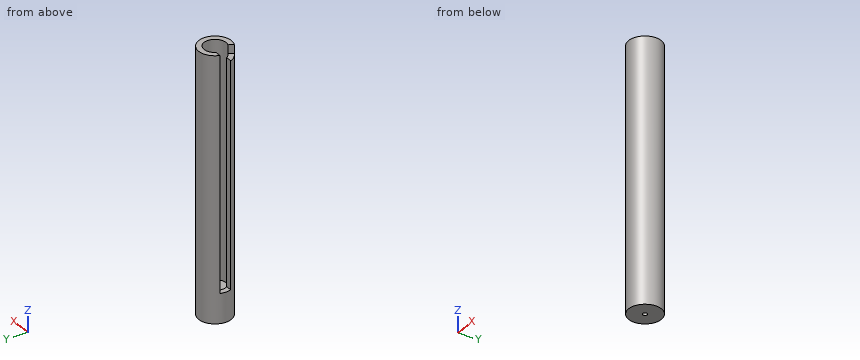
from build123d import *

# Parameters (mm, degrees)
SKETCH1_R           = 19.05
BOSS_EXTRUDE1_DEPTH = 304.8
SKETCH3_R           = 12.7
CUT_EXTRUDE1_DEPTH  = 273.05
SKETCH4_R           = 2.54
CUT_EXTRUDE2_DEPTH  = 31.75
CUT_EXTRUDE3_DEPTH  = 273.05
CUT_EXTRUDE4_DEPTH  = 12.7


with BuildPart() as part:
    # Sketch1 → Boss-Extrude1 (new body)
    with BuildSketch(Plane.XY):
        Circle(SKETCH1_R)
    extrude(amount=BOSS_EXTRUDE1_DEPTH)

    # Sketch3 → Cut-Extrude1 (cut)
    with BuildSketch(Plane.XY.offset(304.8)):
        Circle(SKETCH3_R)
    extrude(amount=-CUT_EXTRUDE1_DEPTH, mode=Mode.SUBTRACT)

    # Sketch4 → Cut-Extrude2 (cut)
    with BuildSketch(Plane(origin=(0, 0, 0), x_dir=(-1, 0, 0), z_dir=(0, 0, -1))):
        Circle(SKETCH4_R)
    extrude(amount=-CUT_EXTRUDE2_DEPTH, mode=Mode.SUBTRACT)

    # Sketch5 → Cut-Extrude3 (cut)
    with BuildSketch(Plane.XY.offset(307.34)):
        Polygon((-12.7, 6.35), (-8.710116392, 6.35), (-8.710116392, -6.35), (-20.268037983, -6.35), (-20.268037983, 6.35), align=None)
    extrude(amount=-CUT_EXTRUDE3_DEPTH, mode=Mode.SUBTRACT)

    # Sketch7 → Cut-Extrude4 (cut)
    with BuildSketch(Plane.XY.offset(307.34)):
        Polygon((-17.960512242, -6.35), (-18.177595791, -12.696288264), (-18.177595791, -17.489691447), (-8.665474889, -17.489691447), (-4.23331347, -9.662232457), (-8.307734332, -6.35), align=None)
    extrude(amount=-CUT_EXTRUDE4_DEPTH, mode=Mode.SUBTRACT)


solid = part.part
For this review, take the finished solid that the model builds, in its own axes (mm). Round coordinates to 2 decimals unless told otherwise and drop trailing zeros. Order: outer loops, then holes, each group sorted by start corner. A loop starts at its lowest first (then second) coordinate and runs counter-clockwise, first axis right, second up. Notation, with made-up numbers: (37.5, 49) -> (54.5, 49) arc R21 cw to (54.5, 68) -> close; hole circle Ø11 at (82, 1). An arc over 180 degrees is marked (long way). Put each result on its own line as item: value.
Q1. Insertion check: pin 1 Ø8 at (x, z) = (9, 227.5) entering from +Y; pin 2 Ø3 at (x, z) = (10.5, 222) entering from +Y; pin 3 Ø12 at (y, z) = (8.5, 39) entering from +X; pin 4 Ø8 at (x, y) = (-9.5, 14.5) entering from -Z. Each pin has a flat end and moves straight along its axis. Give the tip position at first contact, or say it passes through.
Check result:
pin 1: y = 18.38
pin 2: y = 16.79
pin 3: x = 18.89
pin 4: z = 0
Q2. Add section B-B on y = 0. Write out the cut boundary in (x, z), plus the area to 3 significant figures.
Check result:
outline: (-19.05, 0) -> (-2.54, 0) -> (-2.54, 31.75) -> (-12.7, 31.75) -> (-12.7, 34.29) -> (-19.05, 34.29) -> close; (2.54, 0) -> (19.05, 0) -> (19.05, 304.8) -> (12.7, 304.8) -> (12.7, 31.75) -> (2.54, 31.75) -> close
area: 2,800 mm2
Q3. Add section C-C on z = 62. Write out the cut boundary in (x, y).
Check result:
outline: (-17.96, -6.35) arc R19.05 ccw (long way) to (-17.96, 6.35) -> (-11, 6.35) arc R12.7 cw (long way) to (-11, -6.35) -> close
Q4. Add section A-A on x = 0. Write out the cut boundary in (y, z), plus the area to 3 significant figures.
Check result:
outline: (-19.05, 0) -> (-2.54, 0) -> (-2.54, 31.75) -> (-12.7, 31.75) -> (-12.7, 304.8) -> (-19.05, 304.8) -> close; (2.54, 0) -> (19.05, 0) -> (19.05, 304.8) -> (12.7, 304.8) -> (12.7, 31.75) -> (2.54, 31.75) -> close
area: 4,520 mm2
Q5. Add section D-D on x = 15.5. Write out the cut boundary in (y, z), plus the area to 3 significant figures.
Check result:
outline: (-11.07, 0) -> (11.07, 0) -> (11.07, 304.8) -> (-11.07, 304.8) -> close
area: 6,750 mm2
Q6. For probe 1 along Y at (x, z) = (0, 8.5); probe 2 along Z at (x, y) = (7, 6); probe 3 along X at (y, z) = (0, 240), list the stretches that pass through material, from the lowest coordinate up. Write a range as [from, to].
Check result:
probe 1: [-19.05, -2.54], [2.54, 19.05]
probe 2: [0, 31.75]
probe 3: [12.7, 19.05]
